from build123d import *

# Parameters (mm, degrees)
SKETCH1_W           = 279.4
SKETCH1_H           = 368.3
BOSS_EXTRUDE1_DEPTH = 101.6
CUT_EXTRUDE2_DEPTH  = 343.662
CUT_EXTRUDE3_DEPTH  = 81.788
FILLET2_R           = 2.38


with BuildPart() as part:
    # Sketch1 → Boss-Extrude1 (new body)
    with BuildSketch(Plane.XY):
        with Locations((65.648946297, -14.210932476)):
            Rectangle(SKETCH1_W, SKETCH1_H)
    extrude(amount=BOSS_EXTRUDE1_DEPTH)

    # Sketch5 → Cut-Extrude2 (cut)
    with BuildSketch(Plane.ZY.offset(74.051053703)):
        Polygon((50.8, 169.939067524), (101.6, 142.764720342), (197.27126928, 191.743775141), (59.221541493, 225.542979991), align=None)
        Polygon((197.27126928, -220.165640093), (59.221541493, -253.964844943), (50.8, -198.360932476), (101.6, -171.186585294), align=None)
    extrude(amount=-CUT_EXTRUDE2_DEPTH, mode=Mode.SUBTRACT)

    # Sketch6 → Cut-Extrude3 (cut)
    with BuildSketch(Plane(origin=(0, -200.900932476, 0), x_dir=(-1, 0, 0), z_dir=(0, -1, 0))):
        with BuildLine():
            Line((47.465898878, -87.350896203), (-178.763791471, -87.350896203))
            ThreePointArc((-178.763791471, -87.350896203), (-188.288791471, -77.825896203), (-178.763791471, -68.300896203))
            Line((-178.763791471, -68.300896203), (47.465898878, -68.300896203))
            ThreePointArc((47.465898878, -68.300896203), (56.990898878, -77.825896203), (47.465898878, -87.350896203))
        make_face()
    extrude(amount=-CUT_EXTRUDE3_DEPTH, mode=Mode.SUBTRACT)

    # Fillet2
    fillet2_edges = [part.edges().sort_by_distance(p)[0] for p in [
        (-74.051053703, -14.210932476, 101.6),
        (205.348946297, -14.210932476, 101.6),
        (65.648946297, -171.186585294, 101.6),
        (65.648946297, 142.764720342, 101.6),
        (-74.051053703, 169.939067524, 25.4),
        (205.348946297, 169.939067524, 25.4),
        (205.348946297, -198.360932476, 25.4),
        (-74.051053703, -198.360932476, 25.4),
        (205.348946297, 156.351893933, 76.2),
        (-74.051053703, 156.351893933, 76.2),
        (65.648946297, 169.939067524, 50.8),
        (205.348946297, -184.773758885, 76.2),
        (65.648946297, -198.360932476, 50.8),
        (-74.051053703, -184.773758885, 76.2),
        (205.348946297, -14.210932476, 0),
        (65.648946297, -198.360932476, 0),
        (-74.051053703, -14.210932476, 0),
    ]]
    fillet(fillet2_edges, radius=FILLET2_R)


solid = part.part
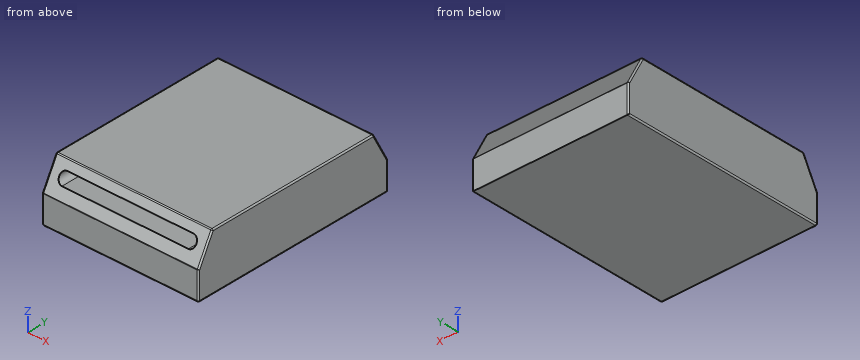
Check sheet for the modelled part. Datum: model origin and axes. Units: mm. Give positions to 0.01 mm unless a question says otherwise; leave off trailing zeros. Loops run counter-clockwise (first coordinate to the right, second up) from the corner with the lowest first, then second, coordinate; pieces in that order, holes last. Notation, with made-up numbers: M 73,17 L 124,17 A24 ccw 124,42 Z; hole C -6.5,33.25 d3. An arc over 180 degrees is marked long. Use a Markdown table: item, result. Add a question column.
Q1. Sectioned sample at B-B, the plane x = 127. Record the cut outline in (y, z).
Q2. Scan lines: line 1 along Z through (x, y) = (-35, -156.5); line 2 along Z through (x, y) = (-31.5, -175.5); line 3 along Y through (x, z) = (-60, 83.5). Record each from-to range of solid material in increasing order. Write a range as [from, to].
Q3. Sectioned sample at A-A, the plane y = -149. Record the cut outline in (x, z) (3 decimals).
Q4. Go/stop test with flat-tipped pins: pin 1 (5.5 mm diameter, centred on x = 65.5, z = 76.5, fed in from -Y); pin 2 (2 mm diameter, centred on x = 81.5, z = 55.5, fed in from -Y). Record where each tip stops, or that it passes through.
Verdict:
| question | item | result |
|---|---|---|
| 1 | outline | M -198.36,2.38 A2.38 ccw -195.98,0 L 169.94,0 L 169.94,50.2 A2.38 ccw 169.66,51.33 L 143.44,100.34 A2.38 ccw 141.34,101.6 L -169.76,101.6 A2.38 ccw -171.86,100.34 L -178.81,87.35 L -119.11,87.35 L -119.11,68.3 L -189,68.3 L -198.08,51.33 A2.38 ccw -198.36,50.2 Z |
| 2 | line 1 | [0, 68.3], [87.35, 101.6] |
| 2 | line 2 | [0, 68.3], [87.35, 93.54] |
| 2 | line 3 | [-180.87, 152.45] |
| 3 | outline | M -74.051,2.38 A2.38 ccw -71.671,0 L 202.969,0 A2.38 ccw 205.349,2.38 L 205.349,99.22 A2.38 ccw 202.969,101.6 L -71.671,101.6 A2.38 ccw -74.051,99.22 Z; hole M -47.466,68.301 L 178.764,68.301 A9.525 ccw 178.764,87.351 L -47.466,87.351 A9.525 ccw Z |
| 4 | pin 1 | y = -119.11 |
| 4 | pin 2 | y = -196.38 |
